Answer from the drawing. Dimensions are ordinates in mm from the lowest x, y and z of the part. A direction names the side the tool comes from. Coordinates: 2 decimals unless noted, no trailing zeros. Order: outer loops, then holes, each group sorted by start corner. A loop starts at its lowest first (then second) coordinate and runs counter-clockwise, first axis right, second up.
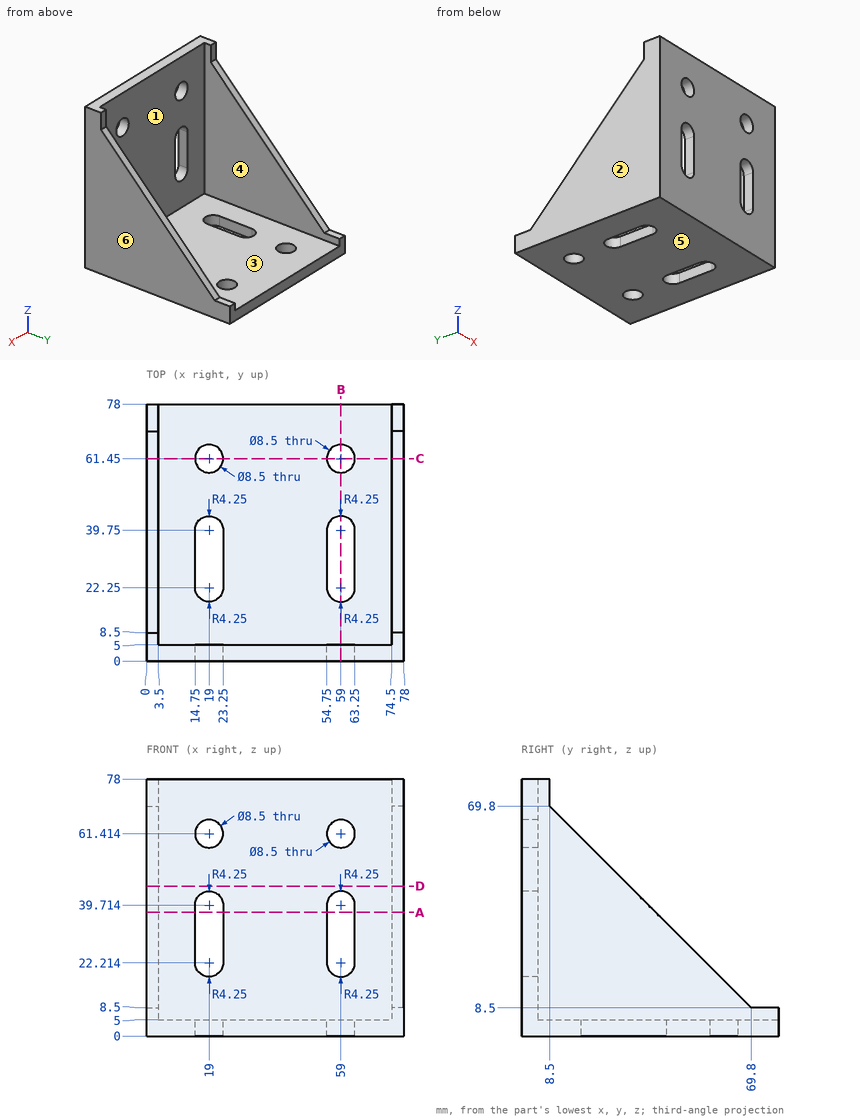
1. The part is cut by section A-A (z = 37.5). Determine the outline of the cut face in (x, y).
2. The part is cut by section B-B (x = 59). Determine the outline of the cut face in (y, z), plus the area to 3 significant figures.
3. Flat-ended cylindrical pins translate along their axes: pin 1 (12 mm diameter, centred on x = 45.5, y = 52, fed in from +Z); pin 2 (2 mm diameter, centred on x = 42.5, z = 59.5, fed in from +Y); pin 3 (3 mm diameter, centred on x = 76, y = 72.5, fed in from +Z); pin 4 (5 mm diameter, centred on x = 59, y = 61.45, fed in from +Z). Find the tip coordinate at first contact, or state that the pin passes through.
4. Consider probe 1 along Y at (x, z) = (19, 2.5); probe 2 along Z at (x, y) = (59, 1.1); probe 3 along X at (y, z) = (44, 17.5). Determine where each line is inside the solid, lowest interval first.
5. For the marked faces 1 and 2, determine the directions among +Z, -Z, +X, -X, +Y, -Y from which every point of the face is accessible in a straight line to the end or side of a thin tool.
6. The mould has two halves that part along X. Classify the marked faces 3, 4, 5 and 6: released by +X, released by -X, zero draft, split by the parting line, or undercut.
7. The part is cut by section D-D (z = 45.5). Determine the outline of the cut face in (x, y).
8. The part is cut by section C-C (y = 61.45). Determine the outline of the cut face in (x, z).
Worked out:
1. outline: (0, 0) - (14.75, 0) - (14.75, 5) - (3.5, 5) - (3.5, 40.8) - (0, 40.8) - close; (23.25, 0) - (54.75, 0) - (54.75, 5) - (23.25, 5) - close; (63.25, 0) - (78, 0) - (78, 40.8) - (74.5, 40.8) - (74.5, 5) - (63.25, 5) - close
2. outline: (0, 0) - (18, 0) - (18, 5) - (5, 5) - (5, 17.96) - (0, 17.96) - close; (0, 43.96) - (5, 43.96) - (5, 57.16) - (0, 57.16) - close; (0, 65.66) - (5, 65.66) - (5, 78) - (0, 78) - close; (44, 0) - (57.2, 0) - (57.2, 5) - (44, 5) - close; (65.7, 0) - (78, 0) - (78, 5) - (65.7, 5) - close
2. area: 410 mm2
3. pin 1: stops at z = 5
3. pin 2: stops at y = 5
3. pin 3: stops at z = 8.5
3. pin 4: passes through
4. probe 1: y = 0 to 18, 44 to 57.2, 65.7 to 78
4. probe 2: z = 0 to 17.96, 43.96 to 57.16, 65.66 to 78
4. probe 3: x = 0 to 3.5, 74.5 to 78
5. face 1: +Z, +Y
5. face 2: +Z, -Z, -X, +Y, -Y
6. face 3: undercut
6. face 4: undercut
6. face 5: zero draft
6. face 6: released by +X
7. outline: (0, 0) - (78, 0) - (78, 32.8) - (74.5, 32.8) - (74.5, 5) - (3.5, 5) - (3.5, 32.8) - (0, 32.8) - close
8. outline: (0, 0) - (14.75, 0) - (14.75, 5) - (3.5, 5) - (3.5, 16.85) - (0, 16.85) - close; (23.25, 0) - (54.75, 0) - (54.75, 5) - (23.25, 5) - close; (63.25, 0) - (78, 0) - (78, 16.85) - (74.5, 16.85) - (74.5, 5) - (63.25, 5) - close
